The drawing under review shows one solid part. Ordinate dimensions are in mm from its lowest x, y, z. Coordinates: 2 decimals unless noted, no trailing zeros. Loops run counter-clockwise (first coordinate to the right, second up) from the corner with the lowest first, then second, coordinate; pieces in that order, holes last. Notation, with made-up numbers: M 67.5,44 L 88.5,44 A7 ccw 88.5,54 Z; hole C 57.25,16.5 d8. An arc over 180 degrees is marked long. Put each result on its own line as item: value.
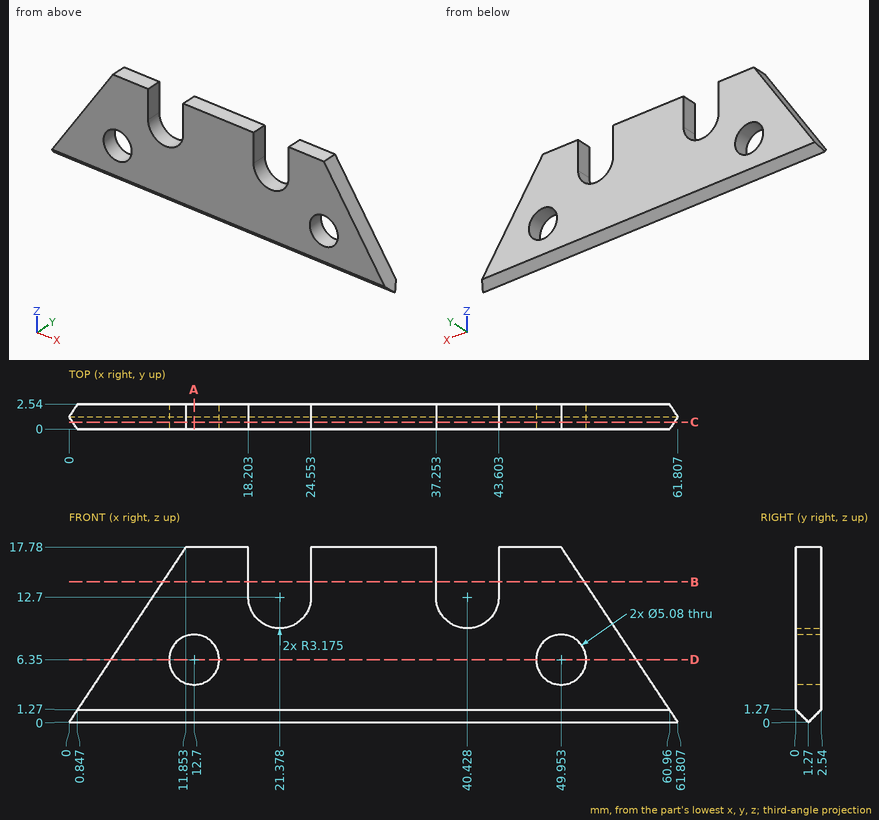
(1) Add section A-A (x = 12.7). Write out the cut boundary in (y, z).
Determined:
outline: M 0,1.27 L 1.27,0 L 2.54,1.27 L 2.54,3.81 L 0,3.81 Z; M 0,8.89 L 2.54,8.89 L 2.54,17.78 L 0,17.78 Z
(2) For pin 1 (1.3 mm diameter, centred on y = 1, z = 15.5, fed in from -X); pin 2 (1 mm diameter, centred on y = 1, z = 8.5, fed in from -X); pin 3 (1.3 mm diameter, centred on y = 1, z = 16, fed in from +X), all flat-tipped, find the tip position at first contact; note any pin that passes through.
Determined:
pin 1: stops at x = 9.9
pin 2: stops at x = 5.33
pin 3: stops at x = 51.57
(3) Add section D-D (z = 6.35). Write out the cut boundary in (x, y), plus the area to 3 significant figures.
Determined:
outline: M 4.23,0 L 10.16,0 L 10.16,2.54 L 4.23,2.54 Z; M 15.24,0 L 47.41,0 L 47.41,2.54 L 15.24,2.54 Z; M 52.49,0 L 57.57,0 L 57.57,2.54 L 52.49,2.54 Z
area: 110 mm^2
(4) Add section C-C (y = 0.7). State how many separate pieces and enclosed holes the cut face has.
Determined:
separate pieces: 1
enclosed holes: 2
(5) Wall thickness on line 1 along X through (y, z) = (0.7, 15.25); line 2 along X through (y, z) = (0.7, 16.5); line 3 along Z through (x, y) = (12.7, 0.65): over which ranges is each line inside the solid? List them lowest first. Write a range as [from, to].
Determined:
line 1: x = [10.17, 18.2], [24.55, 37.25], [43.6, 51.64]
line 2: x = [11, 18.2], [24.55, 37.25], [43.6, 50.81]
line 3: z = [0.62, 3.81], [8.89, 17.78]
(6) Add section B-B (z = 14.25). Write out the cut boundary in (x, y).
Determined:
outline: M 9.5,0 L 18.2,0 L 18.2,2.54 L 9.5,2.54 Z; M 24.55,0 L 37.25,0 L 37.25,2.54 L 24.55,2.54 Z; M 43.6,0 L 52.31,0 L 52.31,2.54 L 43.6,2.54 Z
